Part model, mm, in its own coordinate system. Face numbers are marked on the shaded views. A direction names the side the tool comes from. Round coordinates to 2 decimals unless told otherwise and drop trailing zeros. Loops run counter-clockwise (first coordinate to the right, second up) from the corner with the lowest first, then second, coordinate; pieces in that order, holes last. Notation, with made-up numbers: M 78.5,65 L 86.5,65 A34 cw 86.5,97 Z; hole C 51,-27.75 d7. An arc over 180 degrees is marked long. Put each result on its own line as item: value. Start each with the question number.
1) Pull direction Z, two halves, no side cores. Call the marked faces 1, 2 and 3: +Z half, -Z half, draft (parallel to the pull), parting line (faces both ways), or undercut.
2) Drop flat-ended pins along their axis: pin 1 Ø4 at (x, z) = (-11.5, -4.5) entering from -Y; pin 2 Ø2.5 at (y, z) = (1.5, -23.5) entering from +X; pin 3 Ø2.5 at (x, y) = (-22.5, 2) entering from -Z; pin 4 Ø3 at (y, z) = (3.5, -13) entering from -X. Give the stop position or say it passes through.
3) Slice it at C-C on y = 0.8. Give the cut face in (x, z), then the cut area to 3 significant figures.
4) Probe line 1 along X through (y, z) = (3.15, 0); line 2 along X through (y, z) = (0.55, 10.5); line 3 along Z through (x, y) = (11, 2.15). List the from-to ranges inside material, lowest first.
5) Slice it at B-B on z = 0. Give the cut face in (x, y), then the cut area to 3 significant figures.
6) Which spindle directions (+Z, -Z, +X, -X, +Y, -Y) get a long thin tool onto all of the face, cutting with end or side? Do the marked faces 4, 5 and 6. Say none if no direction does.
7) Slice it at D-D on x = 17. Give the cut face in (y, z).
8) Slice it at A-A on x = 0. Give the cut face in (y, z), then the cut area to 3 significant figures.
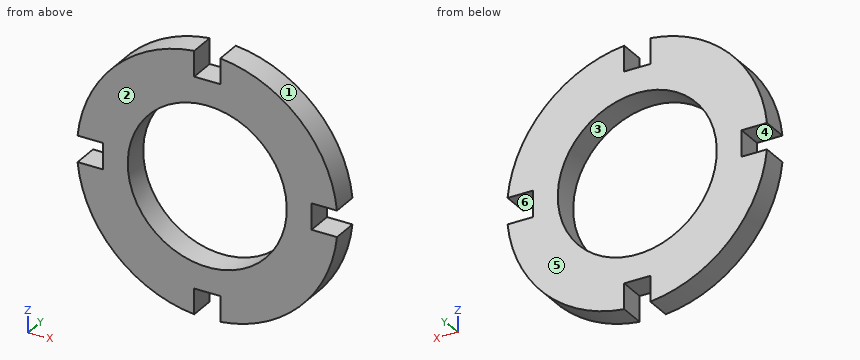
```python
from build123d import *

# Parameters (mm, degrees)
SKETCH1_R           = 25.4
BOSS_EXTRUDE1_DEPTH = 5.08
SKETCH2_R           = 15.494
CUT_EXTRUDE1_DEPTH  = 50.8
SKETCH3_W           = 5.08
SKETCH3_H           = 10.16
CUT_EXTRUDE2_DEPTH  = 50.8
CIRPATTERN1_COUNT   = 4


with BuildPart() as part:
    # Sketch1 → Boss-Extrude1 (new body)
    with BuildSketch(Plane(origin=(0, 0, 0), x_dir=(1, 0, 0), z_dir=(0, 1, 0))):
        with Locations(Location((0, 0, 0), (0, 0, 270))):
            Circle(SKETCH1_R)
    extrude(amount=BOSS_EXTRUDE1_DEPTH)

    # Sketch2 → Cut-Extrude1 (cut)
    with BuildSketch(Plane(origin=(0, 5.08, 0), x_dir=(1, 0, 0), z_dir=(0, 1, 0))):
        with Locations(Location((0, 0, 0), (0, 0, 270))):
            Circle(SKETCH2_R)
    extrude(amount=-CUT_EXTRUDE1_DEPTH, mode=Mode.SUBTRACT)

    # Sketch3 → Cut-Extrude2 (cut)
    with BuildSketch(Plane.XZ):
        with Locations((0, -25.4)):
            Rectangle(SKETCH3_W, SKETCH3_H)
    cut_extrude2 = extrude(amount=-CUT_EXTRUDE2_DEPTH, mode=Mode.SUBTRACT)

    # CirPattern1: Cut-Extrude2 ×4 about axis
    cirpattern1_axis = Axis((0, 0, 0), (0, 1, 0))
    for i in range(1, CIRPATTERN1_COUNT):
        add(cut_extrude2.rotate(cirpattern1_axis, i * 360 / CIRPATTERN1_COUNT), mode=Mode.SUBTRACT)


solid = part.part
```
Recorded:
1. face 1: +Z half
1. face 2: draft
1. face 3: undercut
2. pin 1: passes through
2. pin 2: stops at x = 12.25
2. pin 3: stops at z = -13.91
2. pin 4: stops at x = -22.65
3. outline: M -25.27,-2.54 A25.4 ccw -2.54,-25.27 L -2.54,-20.32 L 2.54,-20.32 L 2.54,-25.27 A25.4 ccw 25.27,-2.54 L 20.32,-2.54 L 20.32,2.54 L 25.27,2.54 A25.4 ccw 2.54,25.27 L 2.54,20.32 L -2.54,20.32 L -2.54,25.27 A25.4 ccw -25.27,2.54 L -20.32,2.54 L -20.32,-2.54 Z; hole C 0,0 d30.99
3. area: 1,170 mm2
4. line 1: x = -20.32 to -15.49, 15.49 to 20.32
4. line 2: x = -23.13 to -11.39, 11.39 to 23.13
4. line 3: z = -22.89 to -10.91, 10.91 to 22.89
5. outline: M -20.32,0 L -15.49,0 L -15.49,5.08 L -20.32,5.08 Z; M 15.49,0 L 20.32,0 L 20.32,5.08 L 15.49,5.08 Z
5. area: 49.0 mm2
6. face 4: -X, +Y, -Y
6. face 5: +Z, -Z, +X, -X, +Y
6. face 6: +X, +Y, -Y
7. outline: M 0,-18.87 L 5.08,-18.87 L 5.08,18.87 L 0,18.87 Z
8. outline: M 0,-20.32 L 5.08,-20.32 L 5.08,-15.49 L 0,-15.49 Z; M 0,15.49 L 5.08,15.49 L 5.08,20.32 L 0,20.32 Z
8. area: 49.0 mm2
